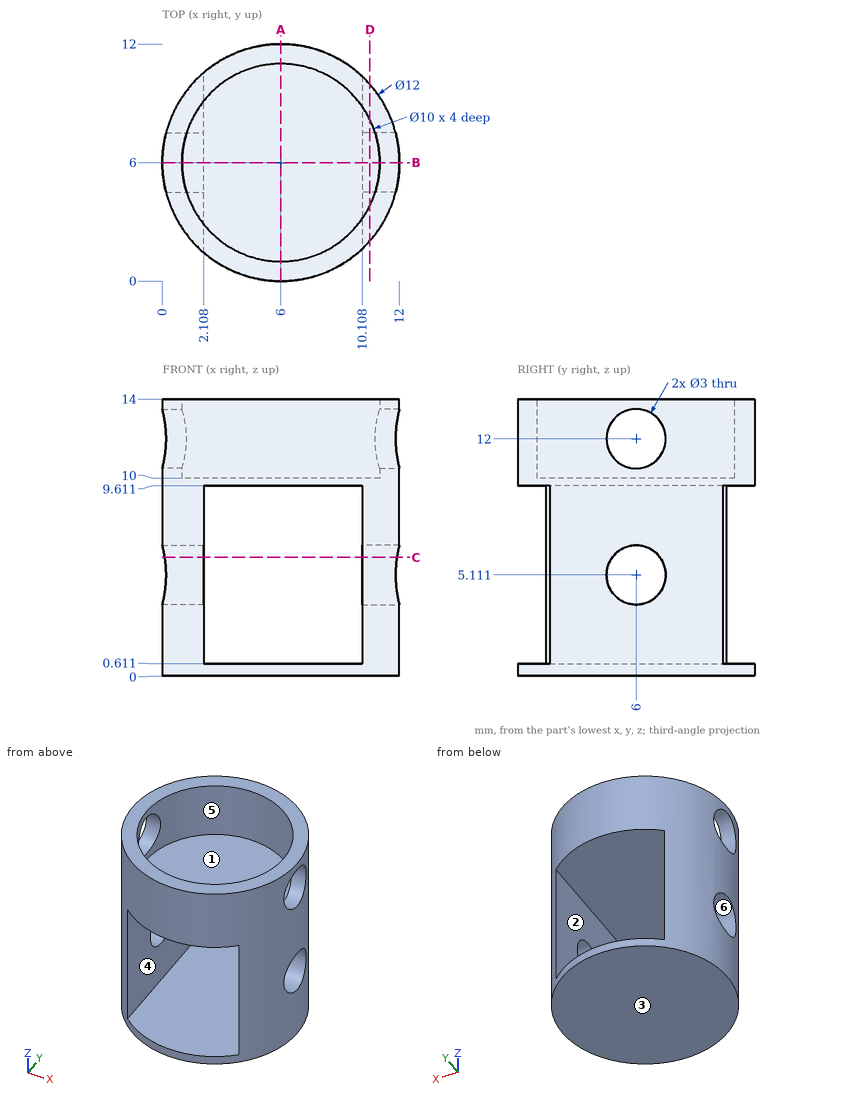
Study the drawing (mm; zero at the part's minimum x, y, z) and answer. A direction names the side the tool comes from. Coordinates: 2 decimals unless noted, no trailing zeros. Loops run counter-clockwise (first coordinate to the right, second up) from the corner with the lowest first, then second, coordinate; pieces in that order, holes last. Notation, with made-up numbers: M 55.25,85.25 L 98.25,85.25 A26 cw 98.25,99.25 Z; hole C 59,77.25 d6. An arc over 180 degrees is marked long. Answer as a JSON object with one key per item and string values. Group by question number.
Item 1: Which of the six approach directions +Z, -Z, +X, -X, +Y, -Y give full straight-line access (tool end or side, diameter ignored) to the marked faces 4, 5 and 6?
Item 2: Determine the mould class of the marked faces 1, 2 and 3 for opening direction Z: +Z half, -Z half, draft (parallel to the pull), parting line (faces both ways), or undercut.
Item 3: Section C-C (z = 6) is taken. Write down the section's boundary in (x, y).
Item 4: Section D-D (x = 10.5) is taken. Write down the section's boundary in (y, z).
Item 5: Each of these flat-tipped pins is pushed along its axis until it touches: P1, Ø1.8, axis at y = 6, z = 12, coming from the +X side; P2, Ø3, axis at x = 4, y = 4, coming from the +Z side. Where does it stop, or does it pass through?
Item 6: Consider L1, parallel to Y at x = 6, z = 11.2; L2, parallel to Z at x = 7, y = 9.75; L3, parallel to Y at x = 11.3, z = 12 (1 decimal). Determine where each line is inside the solid, lowest interval first.
Item 7: Section A-A (x = 6) is taken. Write down the section's boundary in (y, z).
Item 8: Section B-B (y = 6) is taken. Write down the section's boundary in (x, z).
Solved:
{
 "1": {"face 4": "+Y, -Y", "face 5": "+Z", "face 6": "+X, -X"},
 "2": {"face 1": "+Z half", "face 2": "undercut", "face 3": "-Z half"},
 "3": {"outline": "M 0.12,4.79 A6 ccw 2.11,1.43 L 2.11,4.79 Z; M 0.12,7.21 L 2.11,7.21 L 2.11,10.57 A6 ccw Z; M 10.11,1.63 A6 ccw 11.88,4.79 L 10.11,4.79 Z; M 10.11,7.21 L 11.88,7.21 A6 ccw 10.11,10.37 Z"},
 "4": {"outline": "M 2.03,0 L 9.97,0 L 9.97,14 L 8.18,14 L 8.18,10 L 3.82,10 L 3.82,14 L 2.03,14 Z; hole C 6,5.11 d3"},
 "5": {"P1": "passes through", "P2": "stops at z = 10"},
 "6": {"L1": "y = 0 to 1, 11 to 12", "L2": "z = 0 to 0.61, 9.61 to 10", "L3": "y = 3.2 to 4.5, 7.5 to 8.8"},
 "7": {"outline": "M 0,0 L 12,0 L 12,0.61 L 0,0.61 Z; M 0,9.61 L 12,9.61 L 12,14 L 11,14 L 11,10 L 1,10 L 1,14 L 0,14 Z"},
 "8": {"outline": "M 0,0 L 12,0 L 12,3.61 L 10.11,3.61 L 10.11,0.61 L 2.11,0.61 L 2.11,3.61 L 0,3.61 Z; M 0,6.61 L 2.11,6.61 L 2.11,9.61 L 10.11,9.61 L 10.11,6.61 L 12,6.61 L 12,10.5 L 11,10.5 L 11,10 L 1,10 L 1,10.5 L 0,10.5 Z; M 0,13.5 L 1,13.5 L 1,14 L 0,14 Z; M 11,13.5 L 12,13.5 L 12,14 L 11,14 Z"}
}
